Here's the drawing with two shaded views (mm, measured from the low corner). I have some questions. A direction names the side the tool comes from. Coordinates: 2 decimals unless noted, no trailing zeros. Loops run counter-clockwise (first coordinate to the right, second up) from the corner with the lowest first, then second, coordinate; pieces in that order, holes last. Notation, with made-up numbers: M 11,-19 L 58,-19 A24 ccw 58,6 Z; hole C 49.5,32 d8. An arc over 180 degrees is marked long. Use one line per item in the form item = value. Start each with the question number.
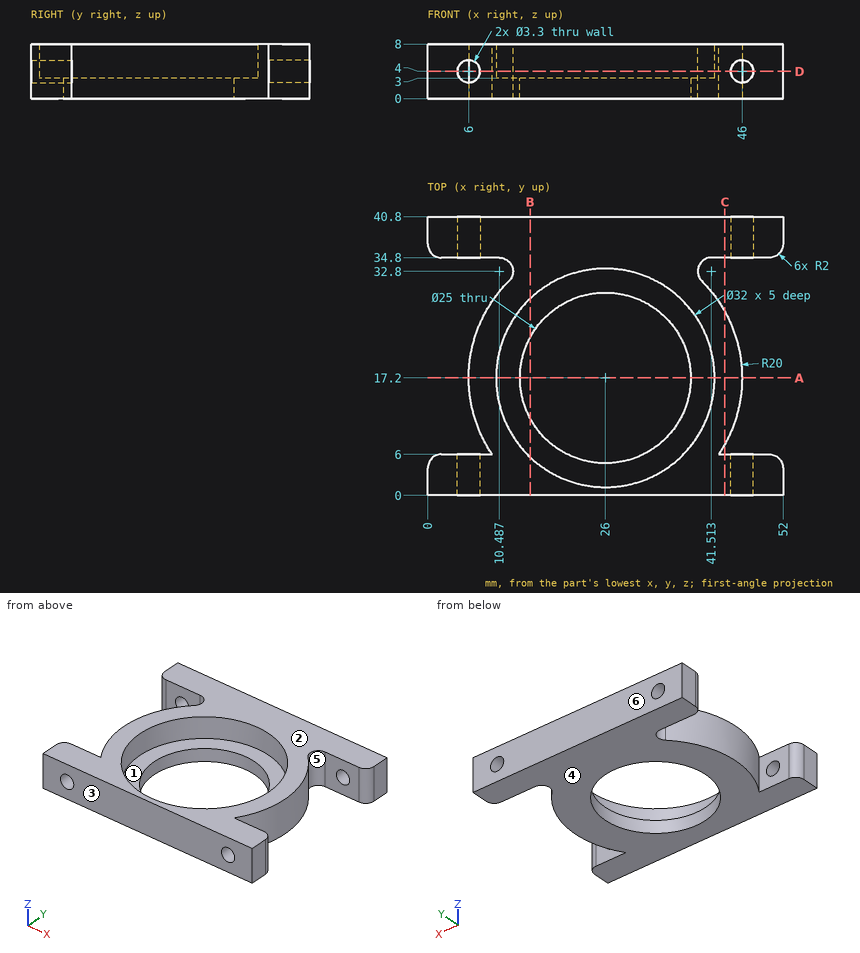
Item 1: Thinking about a two-plate mould opening in Y: for the marked faces 3, 4, 5 and 6, which applies, pulls with the +Y half, pulls with the -Y half, needs draft (parallel to the pull), parting line crosses it, or undercut?
Item 2: I want a section at A-A (y = 17.2). Write out the boundary of the cut face in (x, z).
Item 3: I want a section at B-B (x = 15). Write out the boundary of the cut face in (y, z).
Item 4: For the marked faces 1 and 2, which set-ups out of +Z, -Z, +X, -X, +Y, -Y let a thin tool reach every point of the face, with its end or its side?
Item 5: I want a section at C-C (x = 43.5). Write out the boundary of the cut face in (y, z), plus the area to 3 significant figures.
Item 6: Please list where these lines run through material, in increasing order: line 1 along X through (y, z) = (36.7, 4); line 2 along Y through (x, z) = (26, 2.15); line 3 along Z through (x, y) = (46, 39.5).
Item 7: I want a section at D-D (z = 4). Count the separate pieces of the cut face and the enclosed holes in it.
Item 8: I'm going to push flat-ended pins straight in: P1, Ø16, axis at x = 29.5, y = 21, coming from the +Z side; P2, Ø3, axis at x = 46, z = 4, coming from the +Y side. Where does each tip first touch, or does it pass through?
Worked answers:
q1.face_3 = pulls with the -Y half
q1.face_4 = needs draft
q1.face_5 = undercut
q1.face_6 = pulls with the +Y half
q2.outline = M 6,0 L 13.5,0 L 13.5,3 L 10,3 L 10,8 L 6,8 Z; M 38.5,0 L 46,0 L 46,8 L 42,8 L 42,3 L 38.5,3 Z
q3.outline = M 0,0 L 11.26,0 L 11.26,3 L 5.58,3 L 5.58,8 L 0,8 Z; M 23.14,0 L 40.8,0 L 40.8,8 L 28.82,8 L 28.82,3 L 23.14,3 Z
q4.face_1 = +Z
q4.face_2 = +Z, +X, -X, +Y, -Y
q5.outline = M 0,0 L 6,0 L 6,8 L 0,8 Z; M 7.52,0 L 26.88,0 L 26.88,8 L 7.52,8 Z; M 34.8,0 L 40.8,0 L 40.8,8 L 34.8,8 Z
q5.area = 251 mm²
q6.line_1 = 0 to 4.35, 7.65 to 44.35, 47.65 to 52
q6.line_2 = 0 to 4.7, 29.7 to 40.8
q6.line_3 = 0 to 2.35, 5.65 to 8
q7.separate_pieces = 5
q7.enclosed_holes = 1
q8.P1 = 3
q8.P2 = 24.8
